Geometry check sheet. Reference: the model listing, model coordinates, mm. Face numbers are marked on the shaded views. A direction names the side the tool comes from. Coordinates: 2 decimals unless noted, no trailing zeros. Order: outer loops, then holes, each group sorted by start corner. A loop starts at its lowest first (then second) coordinate and runs counter-clockwise, first axis right, second up. Notation, with made-up numbers: (48.25, 38) - (76.25, 38) arc R21 cw to (76.25, 68) - close; hole circle Ø3 at (-24, 61). An arc over 180 degrees is marked (long way). Use CSV: the item, a comma, the result in double quotes. Start each with the question number.
1) Sectioned sample at A-A, the plane z = 18. Record the cut outline in (x, y).
2) Draft check along Z on the marked faces 5, 6, 7 and 8. Enter one of: released by +Z, released by -Z, zero draft, split by the parting line, or undercut.
3) Sectioned sample at C-C, the plane x = 0. Record the cut outline in (y, z), and give its area (3 significant figures).
4) Depth check by flat-ended pin: P1, Ø3.5, axis at x = -0.5, z = 39.5, coming from the +Y side; P2, Ø2, axis at x = -13.5, y = 2.5, coming from the +Z side; P3, Ø10, axis at y = -8.5, z = 26, coming from the -X side. Enter the tip coordinate at first touch or a pass-through.
5) Tool access check on the marked faces 1, 2, 3 and 4. Record the directions out of +Z, -Z, +X, -X, +Y, -Y that give a thin tool (end or side, any length) a straight path to the whole face; none if there is none.
6) Thickness scan on probe 1 along Y at (x, z) = (15.5, 15); probe 2 along Y at (x, z) = (-15, 18). Record the ranges inside material, lowest first. Write a range as [from, to].
7) Sectioned sample at D-D, the plane y = -3.5. Record the cut outline in (x, z).
8) Sectioned sample at B-B, the plane z = 0. Record the cut outline in (x, y).
from build123d import *

# Parameters (mm, degrees)
F0_W      = 42.3
F0_H      = 42.3
F1_DEPTH  = 10
F2_SIZE   = 7.62
F3_W      = 42.418
F3_H      = 42.418
F4_DEPTH  = 10
F5_SIZE   = 5.08
F7_DEPTH  = 10
F8_R      = 10.9982
F9_DEPTH  = 2
F10_R     = 2.5
F11_DEPTH = 22
F13_DEPTH = 15
F14_R     = 1.5
F15_DEPTH = 6.35


with BuildPart() as f1:
    # F0 (on Top) → F1 (new body, symmetric)
    with BuildSketch(Plane.XY):
        Rectangle(F0_W, F0_H)
    extrude(amount=F1_DEPTH, both=True)

    # F2
    f2_edges = [f1.edges().sort_by_distance(p)[0] for p in [
        (21.15, 21.15, 0),
        (-21.15, 21.15, 0),
        (-21.15, -21.15, 0),
        (21.15, -21.15, 0),
    ]]
    chamfer(f2_edges, length=F2_SIZE)

    # F3 (on face) → F4 (join)
    with BuildSketch(Plane.XY.offset(10)):
        Rectangle(F3_W, F3_H)
        Polygon((-13.53, 21.15), (13.53, 21.15), (21.15, 13.53), (21.15, -13.53), (13.53, -21.15), (-13.53, -21.15), (-21.15, -13.53), (-21.15, 13.53), align=None, mode=Mode.SUBTRACT)
        Polygon((21.15, 13.53), (13.53, 21.15), (-13.53, 21.15), (-21.15, 13.53), (-21.15, -13.53), (-13.53, -21.15), (13.53, -21.15), (21.15, -13.53), align=None)
    extrude(amount=F4_DEPTH)

    # F5
    f5_edges = [f1.edges().sort_by_distance(p)[0] for p in [
        (21.209, 21.209, 15),
        (-21.209, 21.209, 15),
        (-21.209, -21.209, 15),
        (21.209, -21.209, 15),
    ]]
    chamfer(f5_edges, length=F5_SIZE)

    # F6 (on face) → F7 (join)
    with BuildSketch(Plane(origin=(0, 0, -10), x_dir=(1, 0, 0), z_dir=(0, 0, -1))):
        Polygon((16.129, 21.209), (-16.129, 21.209), (-21.209, 16.129), (-21.209, -16.129), (-16.129, -21.209), (16.129, -21.209), (21.209, -16.129), (21.209, 16.129), align=None)
        Polygon((13.53, -21.15), (-13.53, -21.15), (-21.15, -13.53), (-21.15, 13.53), (-13.53, 21.15), (13.53, 21.15), (21.15, 13.53), (21.15, -13.53), align=None, mode=Mode.SUBTRACT)
        Polygon((-21.15, -13.53), (-13.53, -21.15), (13.53, -21.15), (21.15, -13.53), (21.15, 13.53), (13.53, 21.15), (-13.53, 21.15), (-21.15, 13.53), align=None)
    extrude(amount=F7_DEPTH)

    # F8 (on face) → F9 (join)
    with BuildSketch(Plane.XY.offset(20)):
        Circle(F8_R)
    extrude(amount=F9_DEPTH)

    # F10 (on face) → F11 (join)
    with BuildSketch(Plane.XY.offset(22)):
        Circle(F10_R)
    extrude(amount=F11_DEPTH)

    # F12 (on face) → F13 (cut)
    with BuildSketch(Plane.XY.offset(44)):
        with BuildLine():
            Line((2.6203631624, 2.9334036984), (-2.6333660554, 2.9334036984))
            Line((-2.6333660554, 2.9334036984), (-2.6333660554, 2))
            Line((-2.6333660554, 2), (-1.5, 2))
            ThreePointArc((-1.5, 2), (0, 2.5), (1.5, 2))
            Line((1.5, 2), (2.6203631624, 2))
            Line((2.6203631624, 2), (2.6203631624, 2.9334036984))
        make_face()
        with BuildLine():
            ThreePointArc((1.5, 2), (0, 2.5), (-1.5, 2))
            Line((-1.5, 2), (1.5, 2))
        make_face()
    extrude(amount=-F13_DEPTH, mode=Mode.SUBTRACT)

    # F14 (on face) → F15 (cut)
    with BuildSketch(Plane.XY.offset(20)):
        with Locations((-15.5, 15.5)):
            Circle(F14_R)
        with Locations((15.5, 15.5)):
            Circle(F14_R)
        with Locations((15.5, -15.5)):
            Circle(F14_R)
        with Locations((-15.5, -15.5)):
            Circle(F14_R)
    extrude(amount=-F15_DEPTH, mode=Mode.SUBTRACT)


solid = f1.part
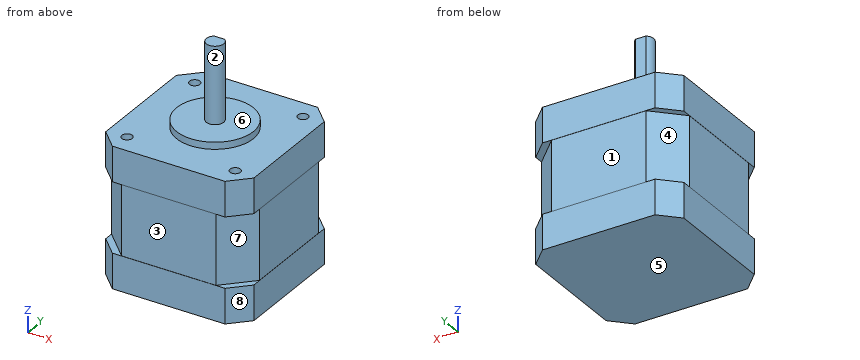
Evaluation:
1,outline,"(-21.21, -16.13) - (-16.13, -21.21) - (16.13, -21.21) - (21.21, -16.13) - (21.21, 16.13) - (16.13, 21.21) - (-16.13, 21.21) - (-21.21, 16.13) - close; hole circle Ø3 at (-15.5, -15.5); hole circle Ø3 at (-15.5, 15.5); hole circle Ø3 at (15.5, -15.5); hole circle Ø3 at (15.5, 15.5)"
2,face 5,"released by -Z"
2,face 6,"released by +Z"
2,face 7,"undercut"
2,face 8,"zero draft"
3,outline,"(-21.21, -20) - (21.21, -20) - (21.21, -10) - (21.15, -10) - (21.15, 10) - (21.21, 10) - (21.21, 20) - (11, 20) - (11, 22) - (2.5, 22) - (2.5, 29) - (2, 29) - (2, 44) - (-2.5, 44) - (-2.5, 22) - (-11, 22) - (-11, 20) - (-21.21, 20) - (-21.21, 10) - (-21.15, 10) - (-21.15, -10) - (-21.21, -10) - close"
3,area,"1,840 mm²"
4,P1,"y = 2"
4,P2,"z = 20"
4,P3,"x = -9.52"
5,face 1,"+X, -X, +Y"
5,face 2,"+Z"
5,face 3,"+X, -X, -Y"
5,face 4,"-X, +Y"
6,probe 1,"[-21.21, -17], [-14, 14], [17, 21.21]"
6,probe 2,"[-21.21, -16.91], [-14.09, 14.09], [16.91, 21.21]"
7,outline,"(-21.21, -20) - (21.21, -20) - (21.21, -10) - (21.15, -10) - (21.15, 10) - (21.21, 10) - (21.21, 20) - (10.43, 20) - (10.43, 22) - (-10.43, 22) - (-10.43, 20) - (-21.21, 20) - (-21.21, 10) - (-21.15, 10) - (-21.15, -10) - (-21.21, -10) - close"
8,outline,"(-21.15, -13.53) - (-13.53, -21.15) - (13.53, -21.15) - (21.15, -13.53) - (21.15, 13.53) - (13.53, 21.15) - (-13.53, 21.15) - (-21.15, 13.53) - close"
